```python
from build123d import *

# Parameters (mm, degrees)
F0_W     = 30
F0_H     = 34
F1_DEPTH = 25.4
F2_R     = 4
F3_DEPTH = 34.001
F4_W     = 19.05
F4_H     = 34
F5_DEPTH = 6.35


with BuildPart() as f1:
    # F0 (on Top) → F1 (new body)
    with BuildSketch(Plane.XY):
        Rectangle(F0_W, F0_H)
    extrude(amount=F1_DEPTH)

    # F2 (on face) → F3 (cut, through all)
    with BuildSketch(Plane.XZ.offset(17)):
        with Locations((0, 8.224509)):
            Circle(F2_R)
    extrude(amount=-F3_DEPTH, mode=Mode.SUBTRACT)

    # F4 (on face) → F5 (cut)
    with BuildSketch(Plane.XY.offset(25.4)):
        Rectangle(F4_W, F4_H)
    extrude(amount=-F5_DEPTH, mode=Mode.SUBTRACT)


solid = f1.part
```
For this review, take the finished solid that the model builds, in its own axes (mm). A direction names the side the tool comes from. Give positions to 0.01 mm unless a question says otherwise; leave off trailing zeros. Loops run counter-clockwise (first coordinate to the right, second up) from the corner with the lowest first, then second, coordinate; pieces in that order, holes last. Notation, with made-up numbers: M 71,0.25 L 78,0.25 A29 cw 78,39.25 Z; hole C -14.5,66 d8. An arc over 180 degrees is marked long. One line per item, written item: value. Start each with the question number.
Q1. Add section D-D (x = 7.5). Give the boundary of the cut face in (y, z).
Q2. Add section B-B (z = 23). Give the boundary of the cut face in (x, y) (3 decimals).
Q3. Draft analysis for pull direction X (two halves, no side actions). For faces 3 (the face through (-0.52, -0.24, 12.19)), 4 (the face through (-9.525, 0, 22)), 5 (the face through (12, 0, 25.4)), 6 (the face through (15, 0, 13)), state which applies: released by +X, released by -X, zero draft, split by the parting line, or undercut.
Q4. Machinability: for faces 1 (the face through (0, 0, 0)), 2 (the face through (0, 0, 19.05)), which of the approach directions +Z, -Z, +X, -X, +Y, -Y give a long, thin tool a straight path to every point of the face, cutting with its end or side? Answer none if there is none.
Q5. Add section A-A (x = 0). Give the boundary of the cut face in (y, z).
Q6. For L1, parallel to Z at x = 0, y = 6.5; L2, parallel to X at y = -2, z = 20 (3 decimals); L3, parallel to X at y = -12.5, z = 8, list the stretches that pass through material, from the lowest coordinate up.
Q7. Clearance check with flat-ended pins moving along their axes: pin 1 Ø5 at (x, y) = (-8.5, -3) entering from +Z; pin 2 Ø1.5 at (x, y) = (-4.5, 4.5) entering from +Z. State where each tip first meets the part, or that it passes through.
Reply:
1. outline: M -17,0 L 17,0 L 17,19.05 L -17,19.05 Z
2. outline: M -15,-17 L -9.525,-17 L -9.525,17 L -15,17 Z; M 9.525,-17 L 15,-17 L 15,17 L 9.525,17 Z
3. face 3: undercut
3. face 4: undercut
3. face 5: zero draft
3. face 6: released by +X
4. face 1: -Z, +X, -X, +Y, -Y
4. face 2: +Z, +Y, -Y
5. outline: M -17,0 L 17,0 L 17,4.22 L -17,4.22 Z; M -17,12.22 L 17,12.22 L 17,19.05 L -17,19.05 Z
6. L1: 0 to 4.22, 12.22 to 19.05
6. L2: -15 to -9.525, 9.525 to 15
6. L3: -15 to -3.99, 3.99 to 15
7. pin 1: z = 25.4
7. pin 2: z = 19.05
